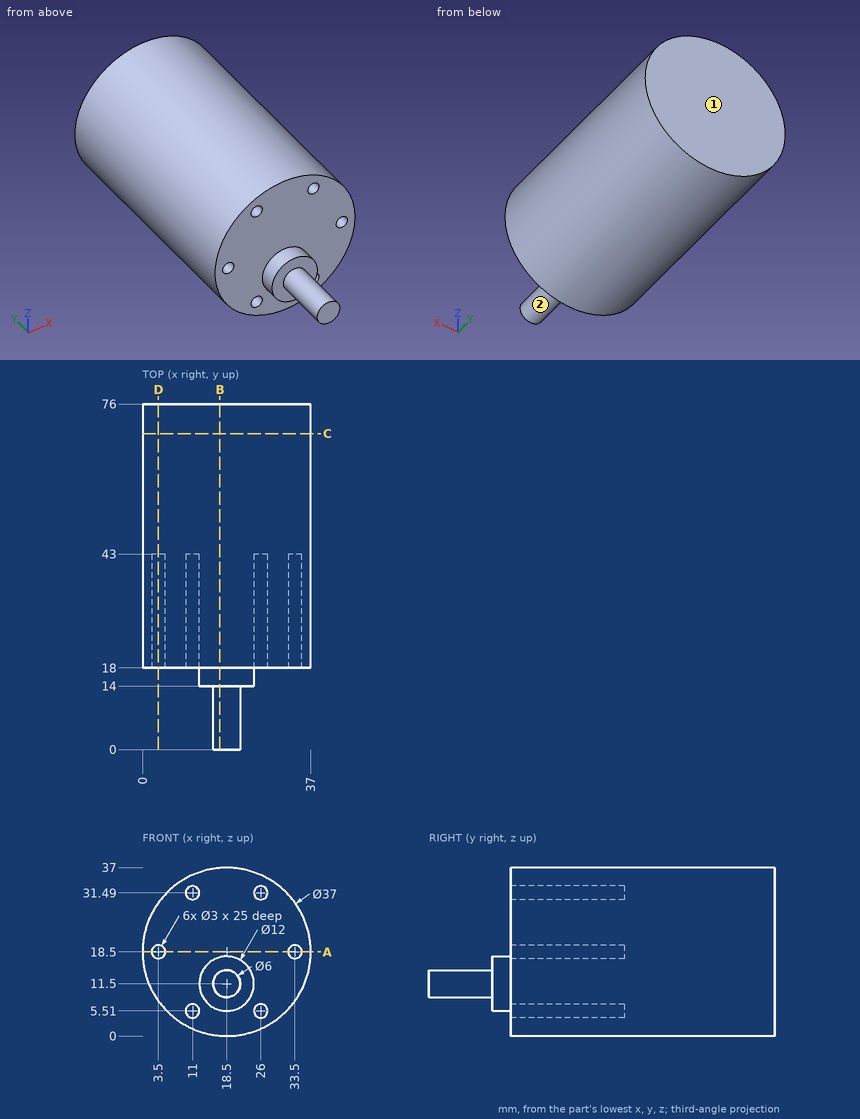
Check sheet for the drawn part. Datum: minimum x, y, z corner. Units: mm. A direction names the side the tool comes from. Round coordinates to 2 decimals unless told otherwise and drop trailing zeros. Write each loop counter-clockwise with the first axis right and the second up, starting at its lowest first coordinate (ties: lowest second). Pieces come first, ordered by that corner, then holes. Notation, with made-up numbers: (-28.5, 4.5) -> (-23.5, 4.5) arc R18 cw to (-23.5, 31.5) -> close; hole circle Ø6 at (41.5, 65.25). An arc over 180 degrees is marked (long way). One line per item, written item: value. Start each with the question number.
(1) Access from +Z, -Z, +X, -X, +Y, -Y to the whole of each face (thin tool, end or side, straight path). Record for the marked faces 1 and 2.
(2) Cross-section at A-A, the plane z = 18.5. Record the cut outline in (x, y).
(3) Cross-section at C-C, the plane y = 69.5. Record the cut outline in (x, z).
(4) Scan lines: line 1 (Z direction, x = 26, y = 25.25); line 2 (Y direction, x = 33, z = 21); line 3 (Z direction, x = 32.5, y = 36) (1 decimal). Record each from-to range of solid material in increasing order. Write a range as [from, to].
(5) Cross-section at D-D, the plane x = 3.5. Record the cut outline in (y, z).
(6) Cross-section at B-B, the plane x = 17. Record the cut outline in (y, z), and give its area (3 significant figures).
(7) Go/stop test with flat-tipped pins: pin 1 Ø3.5 at (x, z) = (19.5, 11.5) entering from -Y; pin 2 Ø3.5 at (x, z) = (11, 5.51) entering from -Y; pin 3 Ø12 at (x, y) = (16, 33.5) entering from -Z; pin 4 Ø0.9 at (x, z) = (25.5, 31) entering from -Y. Record where each tip stops, or that it passes through.
Answer:
1. face 1: +Z, -Z, +X, -X, +Y
1. face 2: -Y
2. outline: (0, 18) -> (2, 18) -> (2, 43) -> (5, 43) -> (5, 18) -> (32, 18) -> (32, 43) -> (35, 43) -> (35, 18) -> (37, 18) -> (37, 76) -> (0, 76) -> close
3. outline: circle Ø37 at (18.5, 18.5)
4. line 1: [1.59, 4.01], [7.01, 29.99], [32.99, 35.41]
4. line 2: [18, 76]
4. line 3: [6.4, 17.4], [19.6, 30.6]
5. outline: (18, 7.67) -> (76, 7.67) -> (76, 29.33) -> (18, 29.33) -> (18, 20) -> (43, 20) -> (43, 17) -> (18, 17) -> close
6. outline: (0, 8.9) -> (14, 8.9) -> (14, 5.69) -> (18, 5.69) -> (18, 0.06) -> (76, 0.06) -> (76, 36.94) -> (18, 36.94) -> (18, 17.31) -> (14, 17.31) -> (14, 14.1) -> (0, 14.1) -> close
6. area: 2,260 mm²
7. pin 1: y = 0
7. pin 2: y = 18
7. pin 3: z = 0
7. pin 4: y = 43
